Could you check a few things on this model? Use its own coordinates, in mm. A direction names the side the tool comes from. Give positions to 0.01 mm unless a question says otherwise; leave off trailing zeros. Loops run counter-clockwise (first coordinate to the right, second up) from the corner with the lowest first, then second, coordinate; pieces in that order, holes last. Notation, with made-up numbers: (-38, 62.25) - (-14, 62.25) arc R17 cw to (-14, 90.25) - close; hole circle Ø4 at (14.25, -32). An arc over 180 degrees is marked (long way). One line per item, written item: value. Start each with the question number.
Q1. I'm going to push flat-ended pins straight in: P1, Ø2, axis at y = -3, z = 11, coming from the -X side; P2, Ø1.5, axis at x = 7, z = 7, coming from the -Y side; P3, Ø3, axis at x = -8.5, y = -0.5, coming from the -Z side; P4, Ø4, axis at x = -6.36, z = -6.36, coming from the +Y side. Where does each tip first touch, or does it pass through?
Q2. If I drill on line 1 (X direction, y = -9, z = -6.25); line 2 (Y direction, x = -7.5, z = -8.5); line 3 (Y direction, x = -5.75, z = -7), over which ranges is the centre line in solid material (lowest first)? Write a range as from..to.
Q3. I want a section at A-A (x = 0). Please give me the cut outline in (y, z), then the cut area to 3 significant figures.
Q4. I want a section at B-B (z = 0). Please give me the cut outline in (x, y).
Q5. I want a section at C-C (y = 8). Please give me the cut outline in (x, z), then the cut area to 3 significant figures.
Q6. If we mould it in two halves opening along Z, with no side actions, what happens to faces 4 (the face through (-6, -6, -6)), 5 (the face through (13.88, 8.75, -1.82)), 6 (the face through (0, 28, 0))? For each: released by +Z, released by -Z, zero draft, split by the parting line, or undercut.
Q7. I want a section at D-D (y = 24.5). Please give me the cut outline in (x, z).
Q8. For faces 1 (the face through (-6, -6, 6)), 2 (the face through (-11, -5, 0)), 3 (the face through (-6, 20, 6)), which set-ups out of +Z, -Z, +X, -X, +Y, -Y let a thin tool reach every point of the face, with its end or its side?
```python
from build123d import *

# Parameters (mm, degrees)
BOSS_EXTRUDE1_DEPTH      = 28
BOSS_EXTRUDE1_DEPTH_BACK = 10
SKETCH1_R                = 14
SKETCH2_R                = 1.5
CUT_EXTRUDE1_DEPTH       = 8
CUT_EXTRUDE2_START       = -4
SKETCH3_R                = 1.5
CUT_EXTRUDE2_DEPTH       = 4
CUT_EXTRUDE3_DEPTH       = 5
SKETCH3_4_R              = 2
BOSS_EXTRUDE2_DEPTH      = 1
CHAMFER1_SIZE            = 1


with BuildPart() as part:
    # Sketch1 → Boss-Extrude1 (new, two sides: drawn at the far end of the back side and taken through both)
    with BuildSketch(Plane(origin=(0, 0, 0), x_dir=(1, 0, 0), z_dir=(0, 1, 0)).offset(-BOSS_EXTRUDE1_DEPTH_BACK)):
        with Locations(Location((0, 0, 0), (0, 0, 270))):
            Circle(SKETCH1_R)
    extrude(amount=BOSS_EXTRUDE1_DEPTH + BOSS_EXTRUDE1_DEPTH_BACK)

    # Sketch2 → Cut-Extrude1 (cut)
    with BuildSketch(Plane(origin=(0, 28, 0), x_dir=(1, 0, 0), z_dir=(0, 1, 0))):
        with Locations(Location((-6.363961031, 6.363961031, 0), (0, 0, 270))):
            Circle(SKETCH2_R)
        with Locations(Location((6.363961031, 6.363961031, 0), (0, 0, 270))):
            Circle(SKETCH2_R)
        with Locations(Location((6.363961031, -6.363961031, 0), (0, 0, 270))):
            Circle(SKETCH2_R)
        with Locations(Location((-6.363961031, -6.363961031, 0), (0, 0, 270))):
            Circle(SKETCH2_R)
    extrude(amount=-CUT_EXTRUDE1_DEPTH, mode=Mode.SUBTRACT)

    # Sketch3 → Cut-Extrude2 (cut)
    with BuildSketch(Plane.XZ.offset(10).offset(CUT_EXTRUDE2_START)):
        with Locations(Location((-6.363961031, 6.363961031, 0), (0, 0, 90))):
            Circle(SKETCH3_R)
        with Locations(Location((6.363961031, 6.363961031, 0), (0, 0, 90))):
            Circle(SKETCH3_R)
        with Locations(Location((-6.363961031, -6.363961031, 0), (0, 0, 90))):
            Circle(SKETCH3_R)
        with Locations(Location((6.363961031, -6.363961031, 0), (0, 0, 90))):
            Circle(SKETCH3_R)
    extrude(amount=CUT_EXTRUDE2_DEPTH, mode=Mode.SUBTRACT)

    # Sketch3_3 → Cut-Extrude3 (cut)
    with BuildSketch(Plane.XZ.offset(10)):
        with BuildLine():
            Line((-8.433766591, 5), (-13.076696831, 5))
            ThreePointArc((-13.076696831, 5), (-14, 0), (-13.076696831, -5))
            Line((-13.076696831, -5), (-8.433766591, -5))
            ThreePointArc((-8.433766591, -5), (-7.726659809, -4.707106781), (-7.433766591, -4))
            Line((-7.433766591, -4), (-7.433766591, 4))
            ThreePointArc((-7.433766591, 4), (-7.726659809, 4.707106781), (-8.433766591, 5))
        make_face()
        with BuildLine():
            Line((-13.076696831, 5), (-20.566233409, 5))
            Line((-20.566233409, 5), (-20.566233409, -5))
            Line((-20.566233409, -5), (-13.076696831, -5))
            ThreePointArc((-13.076696831, -5), (-14, 0), (-13.076696831, 5))
        make_face()
    extrude(amount=-CUT_EXTRUDE3_DEPTH, mode=Mode.SUBTRACT)

    # Sketch3_4 → Boss-Extrude2 (add)
    with BuildSketch(Plane.XZ.offset(10)):
        with Locations(Location((0, 0, 0), (0, 0, 90))):
            Circle(SKETCH3_4_R)
    extrude(amount=BOSS_EXTRUDE2_DEPTH)

    # Chamfer1
    chamfer1_edges = [part.edges().sort_by_distance(p)[0] for p in [
        (0, 28, -14),
        (11.532562595, -10, -7.937253933),
    ]]
    chamfer(chamfer1_edges, length=CHAMFER1_SIZE)


solid = part.part
```
Worked answers:
1. P1: stops at x = -9.8
1. P2: stops at y = -10
1. P3: stops at z = -12.12
1. P4: stops at y = 28
2. line 1: x = -12.53..-7.86, -4.87..4.87, 7.86..12.53
2. line 2: y = -10..28
2. line 3: y = -6..20
3. outline: (-11, -2) - (-10, -2) - (-10, -13) - (-9, -14) - (27, -14) - (28, -13) - (28, 13) - (27, 14) - (-9, 14) - (-10, 13) - (-10, 2) - (-11, 2) - close
3. area: 1,070 mm²
4. outline: (-14, -5) - (-7.43, -5) - (-7.43, -10) - (-2, -10) - (-2, -11) - (2, -11) - (2, -10) - (13, -10) - (14, -9) - (14, 27) - (13, 28) - (-13, 28) - (-14, 27) - close
5. outline: circle Ø28 at (0, 0)
5. area: 616 mm²
6. face 4: undercut
6. face 5: split by the parting line
6. face 6: zero draft
7. outline: circle Ø28 at (0, 0); hole circle Ø3 at (-6.36, -6.36); hole circle Ø3 at (-6.36, 6.36); hole circle Ø3 at (6.36, -6.36); hole circle Ø3 at (6.36, 6.36)
8. face 1: -Y
8. face 2: -X, -Y
8. face 3: +Y
